Part model, mm, in its own coordinate system. A direction names the side the tool comes from. Round coordinates to 2 decimals unless told otherwise and drop trailing zeros. Write each loop counter-clockwise with the first axis right and the second up, starting at its lowest first coordinate (ties: lowest second). Pieces come first, ordered by that corner, then holes. Notation, with made-up numbers: M 43.5,85 L 86.5,85 A21 cw 86.5,111 Z; hole C 85,41.5 d8. An arc over 180 degrees is marked long. Use a Markdown table: item, result. Add a question column.
1) Slice it at C-C on y = 88. Write the cut outline in (x, z).
2) Drop flat-ended pins along their axis: P1, Ø1.5, axis at y = 144, z = 6, coming from the +X side; P2, Ø1.5, axis at x = -1, y = 188.5, coming from the -Z side; P3, Ø1.5, axis at y = 90, z = -3.5, coming from the -X side. Give the stop position or say it passes through.
3) Slice it at B-B on x = 5.75. Write the cut outline in (y, z).
4) Which spindle directions (+Z, -Z, +X, -X, +Y, -Y) get a long thin tool onto all of the face, cutting with end or side? Do faces 1 (the face through (-9.1, 20, -1.4)), 2 (the face through (9.1, 20, 1.3)), 3 (the face through (0, 220, 0)), 4 (the face through (0, 14, -9)), 5 (the face through (-1.172, 118.6, -8.923)). Say none if no direction does.
5) Slice it at A-A on z = 0. Write the cut outline in (x, y).
6) Wall check: probe 1 along Y at (x, z) = (-1.5, 0.5); probe 2 along X at (y, z) = (61, 0.5); probe 3 along X at (y, z) = (90, 4.5). Give the ranges that are in metal, low to high.
```python
from build123d import *

# Parameters (mm, degrees)
SKETCH_1_W          = 20
SKETCH_1_H          = 18
EXTRUDE_1_DEPTH     = 20
SKETCH_2_R          = 9
EXTRUDE_2_DEPTH     = 200
CUT_EXTRUDE_1_DEPTH = 100


with BuildPart() as part:
    # 草图1 → 凸台-拉伸1 (new body)
    with BuildSketch(Plane(origin=(0, 0, 0), x_dir=(1, 0, 0), z_dir=(0, 1, 0))):
        Rectangle(SKETCH_1_W, SKETCH_1_H)
    extrude(amount=EXTRUDE_1_DEPTH)

    # 草图2 → 凸台-拉伸2 (add)
    with BuildSketch(Plane(origin=(0, 20, 0), x_dir=(1, 0, 0), z_dir=(0, 1, 0))):
        Circle(SKETCH_2_R)
    extrude(amount=EXTRUDE_2_DEPTH)

    # 草图3 → 切除-拉伸1 (cut)
    with BuildSketch(Plane.ZY.offset(10)):
        with BuildLine():
            Line((-9, 9), (-9, -3.669557505))
            Line((-9, -3.669557505), (9, -3.669557505))
            Line((9, -3.669557505), (9, 9))
            ThreePointArc((9, 9), (0, 0), (-9, 9))
        make_face()
    extrude(amount=-CUT_EXTRUDE_1_DEPTH, mode=Mode.SUBTRACT)


solid = part.part
```
Entries:
| question | item | result |
|---|---|---|
| 1 | outline | C 0,0 d18 |
| 2 | P1 | stops at x = 7.31 |
| 2 | P2 | stops at z = -9 |
| 2 | P3 | stops at x = -8.57 |
| 3 | outline | M 9,-9 L 20,-9 L 20,-6.92 L 220,-6.92 L 220,6.92 L 20,6.92 L 20,9 L 9,9 A9 ccw Z |
| 4 | face 1 | -X, +Y |
| 4 | face 2 | +X, +Y |
| 4 | face 3 | +Z, -Z, +X, -X, +Y |
| 4 | face 4 | -Z, +X, -X, +Y, -Y |
| 4 | face 5 | +Y |
| 5 | outline | M -10,0 L 10,0 L 10,20 L 9,20 L 9,220 L -9,220 L -9,20 L -10,20 Z |
| 6 | probe 1 | y = 0.01 to 220 |
| 6 | probe 2 | x = -8.99 to 8.99 |
| 6 | probe 3 | x = -7.79 to 7.79 |
